Check sheet for the modelled part. Datum: model origin and axes. Units: mm. A direction names the side the tool comes from. Round coordinates to 2 decimals unless told otherwise and drop trailing zeros. Loops run counter-clockwise (first coordinate to the right, second up) from the corner with the lowest first, then second, coordinate; pieces in that order, holes last. Notation, with made-up numbers: (-3, 7.5) - (17, 7.5) arc R22 cw to (17, 16.5) - close; hole circle Ø4 at (-10, 53). An arc over 180 degrees is marked (long way). Put each result on its own line as item: value.
```python
from build123d import *

# Parameters (mm, degrees)
F0_W     = 14.9
F0_H     = 14.9
F0_R     = 2
F1_DEPTH = 10
F2_DEPTH = 12
F3_W     = 11.7
F3_H     = 11.7
F3_R     = 3.25
F3_R_2   = 2.8
F4_DEPTH = 9


with BuildPart() as f1:
    # F0 (on Top) → F1 (new body)
    with BuildSketch(Plane.XY):
        Rectangle(F0_W, F0_H)
        with Locations((-3.95, -3.95)):
            Circle(F0_R, mode=Mode.SUBTRACT)
        with Locations((3.95, -3.95)):
            Circle(F0_R, mode=Mode.SUBTRACT)
        with Locations((-3.95, 3.95)):
            Circle(F0_R, mode=Mode.SUBTRACT)
        with Locations((3.95, 3.95)):
            Circle(F0_R, mode=Mode.SUBTRACT)
    extrude(amount=F1_DEPTH)

    # F0 (on Top) → F2 (join)
    with BuildSketch(Plane.XY):
        with Locations((-3.95, -3.95)):
            Circle(F0_R)
        with Locations((-3.95, 3.95)):
            Circle(F0_R)
        with Locations((3.95, 3.95)):
            Circle(F0_R)
        with Locations((3.95, -3.95)):
            Circle(F0_R)
    extrude(amount=F2_DEPTH)

    # F3 (on face) → F4 (cut)
    with BuildSketch(Plane(origin=(0, 0, 0), x_dir=(1, 0, 0), z_dir=(0, 0, -1))):
        Rectangle(F3_W, F3_H)
        Circle(F3_R, mode=Mode.SUBTRACT)
        Circle(F3_R_2)
    extrude(amount=-F4_DEPTH, mode=Mode.SUBTRACT)


solid = f1.part
```
Item 1: Section check A-A on z = 1.25. Enter the section's corners in (x, y).
Filled sheet:
outline: (-7.45, -7.45) - (7.45, -7.45) - (7.45, 7.45) - (-7.45, 7.45) - close; circle Ø6.5 at (0, 0); hole (-5.85, -5.85) - (5.85, -5.85) - (5.85, 5.85) - (-5.85, 5.85) - close; hole circle Ø5.6 at (0, 0)
Item 2: Tool access check on faces 1 (the flat face through (-4, 4, 12)), 2 (the flat face through (-5.85, 0, 4)). Record the directions out of +Z, -Z, +X, -X, +Y, -Y that give a thin tool (end or side, any length) a straight path to the whole face; none if there is none.
Filled sheet:
face 1: +Z, +X, -X, +Y, -Y
face 2: -Z
Item 3: Thickness scan on line 1 (Y direction, x = 0, z = 7.25); line 2 (X direction, y = 4.5, z = 7.75). Record the ranges inside material, lowest first. Write a range as from..to.
Filled sheet:
line 1: -7.45..-5.85, -3.25..-2.8, 2.8..3.25, 5.85..7.45
line 2: -7.45..-5.85, 5.85..7.45
Item 4: Section check B-B on x = -3.95. Enter the section's corners in (y, z).
Filled sheet:
outline: (-7.45, 0) - (-5.85, 0) - (-5.85, 9) - (5.85, 9) - (5.85, 0) - (7.45, 0) - (7.45, 10) - (5.95, 10) - (5.95, 12) - (1.95, 12) - (1.95, 10) - (-1.95, 10) - (-1.95, 12) - (-5.95, 12) - (-5.95, 10) - (-7.45, 10) - close
Item 5: Release check for a two-part mould opening along X. For faces 3 (the flat face through (7.45, 0, 5)), 4 (the flat face through (7, 0, 0)), 5 (the cylindrical face through (4.873, -5.724, 10.986)) record: +X half, -X half, draft (parallel to the pull), parting line (faces both ways), or undercut.
Filled sheet:
face 3: +X half
face 4: draft
face 5: undercut
Item 6: Go/stop test with flat-tipped pins: pin 1 (1.5 mm diameter, centred on x = -2.5, y = -1, fed in from +Z); pin 2 (3.5 mm diameter, centred on x = 0, y = 0, fed in from -Z). Record where each tip stops, or that it passes through.
Filled sheet:
pin 1: z = 10
pin 2: z = 9
